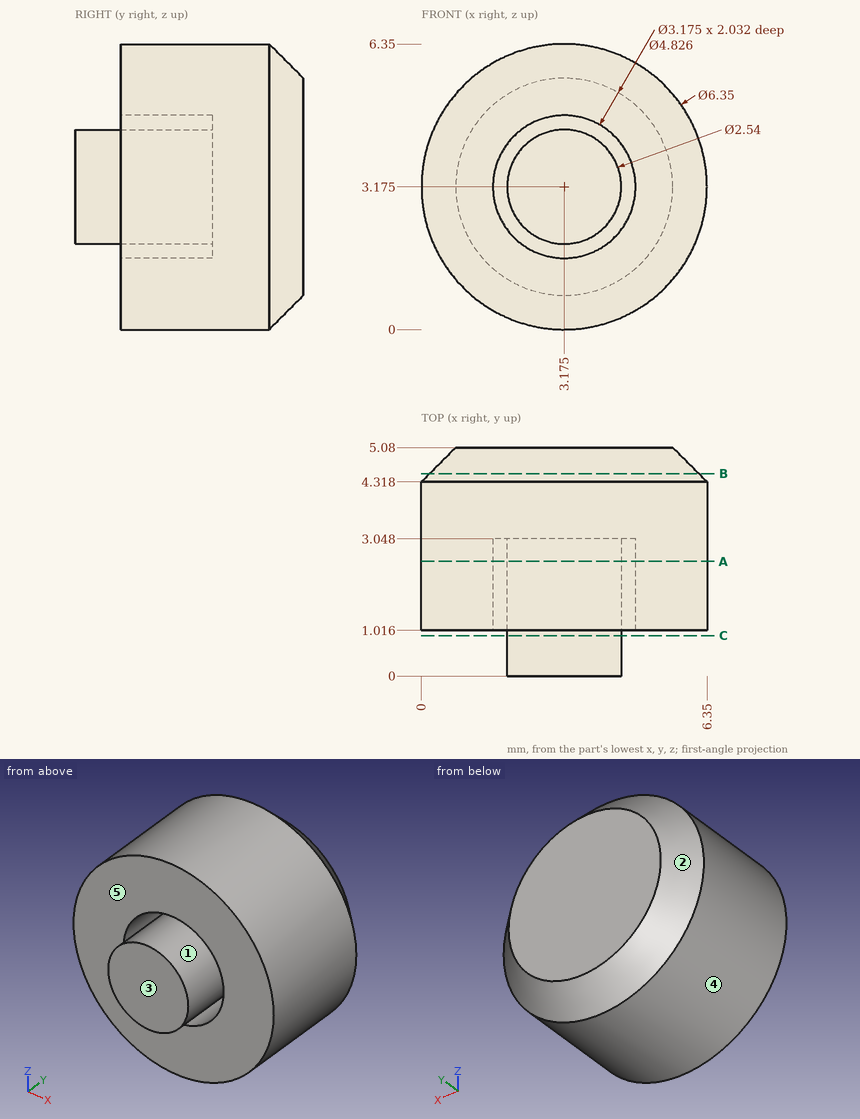
Answer from the drawing. Dimensions are ordinates in mm from the lowest x, y and z of the part. A direction names the side the tool comes from. Give positions to 0.01 mm unless a question says otherwise; leave off trailing zeros. Order: outer loops, then holes, each group sorted by start corner. A loop starts at its lowest first (then second) coordinate and runs counter-clockwise, first axis right, second up.
(1) Given pin 1 (2 mm diameter, centred on x = 2, y = 1.5, fed in from -Z); pin 2 (1 mm diameter, centred on x = 5.5, z = 5.5, fed in from -Y); pin 3 (2 mm diameter, centred on x = 5.5, z = 4.5, fed in from +Y), each flat-ended and moving along its own axis, determine where each tip first touches the part or whether it passes through.
(2) For a pull along Z with two mould halves and no side action, classify the marked faces 1, 2 and 3 as released by +Z, released by -Z, zero draft, split by the parting line, or undercut.
(3) Find section A-A (y = 2.55). Give the number of separate pieces and of enclosed holes in the cut face, plus the area to 3 significant figures.
(4) Find section C-C (y = 0.9). Give the vertices of the cut face in (x, z) (3 decimals), plus the area to 3 significant figures.
(5) For the marked faces 4 and 5, determine the directions among +Z, -Z, +X, -X, +Y, -Y from which every point of the face is accessible in a straight line to the end or side of a thin tool.
(6) Straight lines are drawn through the part: L1, parallel to X at y = 1.9, z = 3.25; L2, parallel to X at y = 1.8, z = 4; L3, parallel to Z at x = 2.25, y = 2.45. For each, find the intervals that lie inside material, in ascending order.
(7) Find section B-B (y = 4.5). Give the vertices of the cut face in (x, z) (3 decimals), plus the area to 3 significant figures.
Result sheet:
1. pin 1: stops at z = 0
1. pin 2: stops at y = 1.02
1. pin 3: stops at y = 5.08
2. face 1: undercut
2. face 2: split by the parting line
2. face 3: zero draft
3. separate pieces: 2
3. enclosed holes: 1
3. area: 28.8 mm2
4. outline: circle Ø2.54 at (3.175, 3.175)
4. area: 5.07 mm2
5. face 4: +Y, -Y
5. face 5: -Y
6. L1: x = 0 to 1.59, 1.91 to 4.44, 4.76 to 6.35
6. L2: x = 0.11 to 1.82, 2.21 to 4.14, 4.53 to 6.24
6. L3: z = 0.14 to 1.88, 2.3 to 4.05, 4.47 to 6.21
7. outline: circle Ø5.986 at (3.175, 3.175)
7. area: 28.1 mm2
